```python
from build123d import *

# Parameters (mm, degrees)
SKETCH1_W           = 130.41
SKETCH1_H           = 75.8
BOSS_EXTRUDE1_DEPTH = 3
SKETCH5_W           = 7.5
SKETCH5_H           = 6
CUT_EXTRUDE4_DEPTH  = 151.868844033
SKETCH6_W           = 7.5
SKETCH6_H           = 6
CUT_EXTRUDE5_DEPTH  = 151.868844033
SKETCH8_R           = 1.025
CUT_EXTRUDE7_DEPTH  = 151.868844033
SKETCH9_R           = 1.025
CUT_EXTRUDE8_DEPTH  = 151.868844033


with BuildPart() as part:
    # Sketch1 → Boss-Extrude1 (new body)
    with BuildSketch(Plane(origin=(0, 0, 0), x_dir=(1, 0, 0), z_dir=(0, 1, 0))):
        with Locations((65.205, -37.9)):
            Rectangle(SKETCH1_W, SKETCH1_H)
    extrude(amount=BOSS_EXTRUDE1_DEPTH)

    # Sketch5 → Cut-Extrude4 (cut, through all)
    with BuildSketch(Plane.XZ):
        with Locations((32.25, 69.8)):
            Rectangle(SKETCH5_W, SKETCH5_H)
        with Locations((19.75, 69.8)):
            Rectangle(SKETCH5_W, SKETCH5_H)
    extrude(amount=-CUT_EXTRUDE4_DEPTH, mode=Mode.SUBTRACT)

    # Sketch6 → Cut-Extrude5 (cut, through all)
    with BuildSketch(Plane.XZ):
        with Locations((98.16, 6)):
            Rectangle(SKETCH6_W, SKETCH6_H)
        with Locations((110.66, 6)):
            Rectangle(SKETCH6_W, SKETCH6_H)
    extrude(amount=-CUT_EXTRUDE5_DEPTH, mode=Mode.SUBTRACT)

    # Sketch8 → Cut-Extrude7 (cut, through all)
    with BuildSketch(Plane.XZ):
        with Locations(Location((120.77, 13.86, 0), (0, 0, 270))):
            Circle(SKETCH8_R)
        with Locations(Location((120.77, 62.86, 0), (0, 0, 270))):
            Circle(SKETCH8_R)
    extrude(amount=-CUT_EXTRUDE7_DEPTH, mode=Mode.SUBTRACT)

    # Sketch9 → Cut-Extrude8 (cut, through all)
    with BuildSketch(Plane.XZ):
        with Locations(Location((62.77, 13.86, 0), (0, 0, 270))):
            Circle(SKETCH9_R)
        with Locations(Location((62.77, 62.86, 0), (0, 0, 270))):
            Circle(SKETCH9_R)
    extrude(amount=-CUT_EXTRUDE8_DEPTH, mode=Mode.SUBTRACT)


solid = part.part
```
Geometry check sheet. Reference: the model listing, model coordinates, mm. A direction names the side the tool comes from. Coordinates: 2 decimals unless noted, no trailing zeros. Write each loop counter-clockwise with the first axis right and the second up, starting at its lowest first coordinate (ties: lowest second). Pieces come first, ordered by that corner, then holes. Notation, with made-up numbers: M 88.25,-39.5 L 92.25,-39.5 A25 cw 92.25,-1.5 Z; hole C -9,-39.5 d7. An arc over 180 degrees is marked long. Answer as a JSON object with one key per item and string values.
1. Draft check along Z on faces 3 (the flat face through (64, 1, 0)), 4 (the flat face through (20, 1, 66.8)), 5 (the flat face through (130.41, 1, 38)). Enter one of: released by +Z, released by -Z, zero draft, split by the parting line, or undercut.
Answers below:
{"face 3": "released by -Z", "face 4": "undercut", "face 5": "zero draft"}
2. Scan lines: L1, parallel to X at y = 1.45, z = 70.5; L2, parallel to Z at x = 120.77, y = 1.9 (3 decimals); L3, parallel to X at y = 1.95, z = 62.86 (3 decimals). Record each from-to range of solid material in increasing order.
Answers below:
{"L1": "x = 0 to 16, 23.5 to 28.5, 36 to 130.41", "L2": "z = 0 to 12.835, 14.885 to 61.835, 63.885 to 75.8", "L3": "x = 0 to 61.745, 63.795 to 119.745, 121.795 to 130.41"}
3. Tool access check on faces 1 (the flat face through (64, 3, 37)), 2 (the flat face through (20, 1, 72.8)). Record the directions out of +Z, -Z, +X, -X, +Y, -Y that give a thin tool (end or side, any length) a straight path to the whole face; none if there is none.
Answers below:
{"face 1": "+Z, -Z, +X, -X, +Y", "face 2": "+Y, -Y"}
4. Section check A-A, the plane y = 0.7. Give the number of separate pieces and of enclosed holes in the cut face, plus the area to 3 significant figures.
Answers below:
{"separate pieces": "1", "enclosed holes": "8", "area": "9,690 mm²"}
5. Section check B-B, the plane x = 111. Enter the section's corners in (y, z), plus the area to 3 significant figures.
Answers below:
{"outline": "M 0,0 L 3,0 L 3,3 L 0,3 Z; M 0,9 L 3,9 L 3,75.8 L 0,75.8 Z", "area": "209 mm²"}
